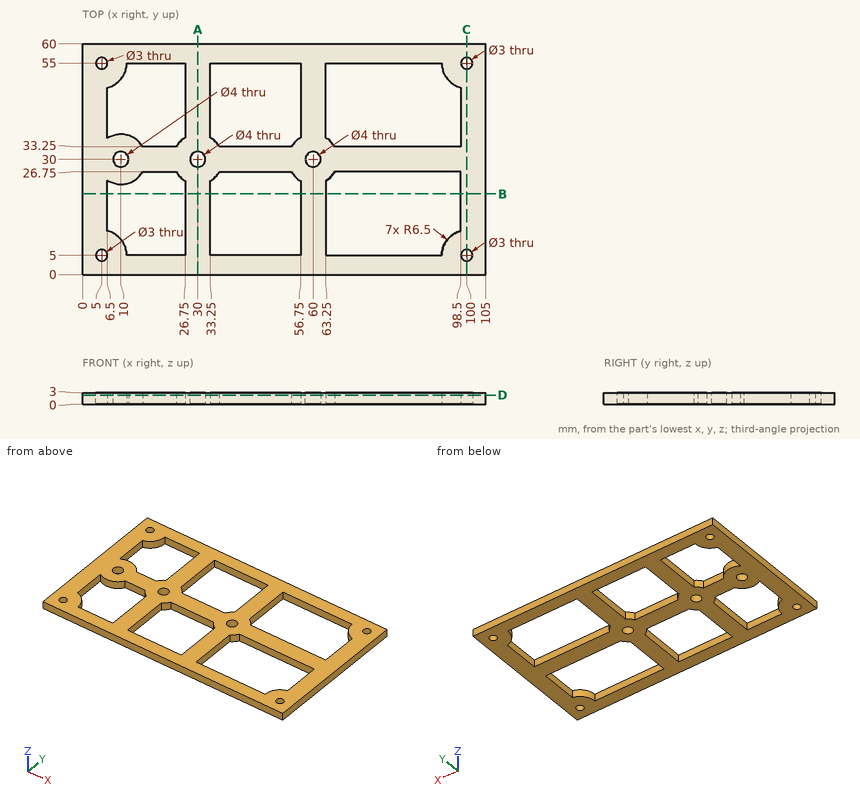
Can you work these out from the drawing? Everything is in mm from the part's minimum corner. Coordinates: 2 decimals unless noted, no trailing zeros. Write each loop counter-clockwise with the first axis right and the second up, starting at its lowest first coordinate (ties: lowest second). Pieces come first, ordered by that corner, then holes. Notation, with made-up numbers: (-1.75, 63.5) -> (43.25, 63.5) arc R21 ccw to (43.25, 72.5) -> close; hole circle Ø1 at (0, -15.75). An arc over 180 degrees is marked (long way). Write each question's results on one line, items separated by ' | '. Start each with the question number.
Q1. Imagine slicing it at C-C (x = 100). Write out the boundary of the cut face in (y, z), then the cut area to 3 significant figures.
Q2. Imagine slicing it at B-B (y = 21). Write out the boundary of the cut face in (x, z).
Q3. Imagine slicing it at D-D (z = 2.35). State how many separate pieces and enclosed holes the cut face has, then the cut area to 3 significant figures.
Q4. Imagine slicing it at A-A (x = 30). Write out the boundary of the cut face in (y, z), then the cut area to 3 significant figures.
Q5. If I drill on probe 1 along X at (y, z) = (48.5, 2.3); probe 2 along Y at (x, z) = (49.5, 2.75); probe 3 along X at (y, z) = (55.5, 0.4), over which ranges is the centre line in solid material (lowest first)?
Taken from the geometry:
1) outline: (0, 0) -> (3.5, 0) -> (3.5, 3) -> (0, 3) -> close; (6.5, 0) -> (53.5, 0) -> (53.5, 3) -> (6.5, 3) -> close; (56.5, 0) -> (60, 0) -> (60, 3) -> (56.5, 3) -> close | area: 162 mm^2
2) outline: (0, 0) -> (6.5, 0) -> (6.5, 3) -> (0, 3) -> close; (26.75, 0) -> (33.25, 0) -> (33.25, 3) -> (26.75, 3) -> close; (56.75, 0) -> (63.25, 0) -> (63.25, 3) -> (56.75, 3) -> close; (98.5, 0) -> (105, 0) -> (105, 3) -> (98.5, 3) -> close
3) separate pieces: 1 | enclosed holes: 13 | area: 2,960 mm^2
4) outline: (0, 0) -> (28, 0) -> (28, 3) -> (0, 3) -> close; (32, 0) -> (60, 0) -> (60, 3) -> (32, 3) -> close | area: 168 mm^2
5) probe 1: x = 0 to 6.5, 26.75 to 33.25, 56.75 to 63.25, 98.5 to 105 | probe 2: y = 0 to 5, 26.75 to 33.25, 55 to 60 | probe 3: x = 0 to 3.59, 6.41 to 98.59, 101.41 to 105
